Part model, mm, in its own coordinate system. A direction names the side the tool comes from. Give positions to 0.01 mm unless a question says otherwise; leave off trailing zeros. Write each loop counter-clockwise with the first axis right and the second up, starting at its lowest first coordinate (ties: lowest second). Pieces come first, ordered by that corner, then holes.
from build123d import *

# Parameters (mm, degrees)
BASE_EXTRUDE_THIN_DEPTH = 4.35
SKETCH2_W               = 1.8
SKETCH2_H               = 4.6
CUT_EXTRUDE1_DEPTH      = 36.373471698


with BuildPart() as part:
    # Sketch1 → Base-Extrude-Thin (new, symmetric)
    with BuildSketch(Plane(origin=(0, 0, 0), x_dir=(1, 0, 0), z_dir=(0, 1, 0))):
        with BuildLine():
            Line((-17.2, -7), (-17.2, -1.5))
            ThreePointArc((-17.2, -1.5), (-16.30105087, 0.420061486), (-14.250691112, 0.959292891))
            Line((-14.250691112, 0.959292891), (-9, 0))
            Line((-9, 0), (9, 0))
            Line((9, 0), (14.250691112, 0.959292891))
            ThreePointArc((14.250691112, 0.959292891), (16.30105087, 0.420061486), (17.2, -1.5))
            Line((17.2, -1.5), (17.2, -7))
            Line((17.2, -7), (16.7, -7))
            Line((16.7, -7), (16.7, -1.5))
            ThreePointArc((16.7, -1.5), (15.980840696, 0.036049189), (14.340552889, 0.467434313))
            Line((14.340552889, 0.467434313), (9.045299693, -0.5))
            Line((9.045299693, -0.5), (-9.045299693, -0.5))
            Line((-9.045299693, -0.5), (-14.340552889, 0.467434313))
            ThreePointArc((-14.340552889, 0.467434313), (-15.980840696, 0.036049189), (-16.7, -1.5))
            Line((-16.7, -1.5), (-16.7, -7))
            Line((-16.7, -7), (-17.2, -7))
        make_face()
    extrude(amount=BASE_EXTRUDE_THIN_DEPTH, both=True)

    # Sketch2 → Cut-Extrude1 (cut, through all)
    with BuildSketch(Plane(origin=(17.2, 0, 0), x_dir=(0, 0, -1), z_dir=(1, 0, 0))):
        with Locations((-4.5, 0)):
            Rectangle(SKETCH2_W, SKETCH2_H)
        with BuildLine():
            Line((-7, 2.35), (-7, -2.35))
            ThreePointArc((-7, -2.35), (-6.414213562, -3.764213562), (-5, -4.35))
            Line((-5, -4.35), (-5, -8))
            Line((-5, -8), (-10, -8))
            Line((-10, -8), (-10, 8))
            Line((-10, 8), (-5, 8))
            Line((-5, 8), (-5, 4.35))
            ThreePointArc((-5, 4.35), (-6.414213562, 3.764213562), (-7, 2.35))
        make_face()
    extrude(amount=-CUT_EXTRUDE1_DEPTH, mode=Mode.SUBTRACT)


solid = part.part
1) Mould opens along X. For faces 4 (the flat face through (-11.662, 0.061, -0.486)), 5 (the flat face through (-17.2, 0, 3)), 6 (the cylindrical face through (-15.962, 0.061, -0.052)), 7 (the flat face through (1.4, -4.35, 0.2)) say: +X half, -X half, draft (parallel to the pull), parting line (faces both ways), or undercut.
Check result:
face 4: undercut
face 5: -X half
face 6: undercut
face 7: draft
2) Saw through at A-A (z = 4). Write the cut outline in (x, y), and give its area (3 significant figures).
Check result:
outline: (-17.2, -4.35) - (-16.7, -4.35) - (-16.7, -2.3) - (-17.2, -2.3) - close; (-17.2, 2.3) - (-16.7, 2.3) - (-16.7, 4.35) - (-17.2, 4.35) - close; (16.7, -4.35) - (17.2, -4.35) - (17.2, -2.3) - (16.7, -2.3) - close; (16.7, 2.3) - (17.2, 2.3) - (17.2, 4.35) - (16.7, 4.35) - close
area: 4.10 mm2
3) Saw through at C-C (z = 2). Write the cut outline in (x, y), and give its area (3 significant figures).
Check result:
outline: (-17.2, -4.35) - (-16.7, -4.35) - (-16.7, 4.35) - (-17.2, 4.35) - close; (16.7, -4.35) - (17.2, -4.35) - (17.2, 4.35) - (16.7, 4.35) - close
area: 8.70 mm2
4) Flat gauge pins, fed straight in: P1, Ø4.5, axis at x = -2.5, y = 0, coming from the +Z side; P2, Ø2.5, axis at x = -2.5, y = 0, coming from the -Z side. Where does each tip first touch, or does it go through?
Check result:
P1: stops at z = 0.5
P2: stops at z = 0
5) Saw through at B-B (y = 0). Write the cut outline in (x, z).
Check result:
outline: (-17.2, 1.5) arc R2.5 ccw to (-14.25, -0.96) - (-9, 0) - (9, 0) - (14.25, -0.96) arc R2.5 ccw to (17.2, 1.5) - (17.2, 3.6) - (16.7, 3.6) - (16.7, 1.5) arc R2 cw to (14.34, -0.47) - (9.05, 0.5) - (-9.05, 0.5) - (-14.34, -0.47) arc R2 cw to (-16.7, 1.5) - (-16.7, 3.6) - (-17.2, 3.6) - close; (-17.2, 5.4) - (-16.7, 5.4) - (-16.7, 7) - (-17.2, 7) - close; (16.7, 5.4) - (17.2, 5.4) - (17.2, 7) - (16.7, 7) - close
6) 3-axis set-ups, long thin cutter, end or side, ignore diameter. For faces 1 (the flat face through (0, 0, 0)), 2 (the flat face through (16.7, 0, 3)), 3 (the flat face through (17.2, 0, 3)): which of +Z, -Z, +X, -X, +Y, -Y reach the whole face in a straight line?
Check result:
face 1: -Z, +Y, -Y
face 2: +Z, +Y, -Y
face 3: +Z, -Z, +X, +Y, -Y
7) Saw through at D-D (z = 6). Write the cut outline in (x, y), and give its area (3 significant figures).
Check result:
outline: (-17.2, -4.08) - (-16.7, -4.08) - (-16.7, 4.08) - (-17.2, 4.08) - close; (16.7, -4.08) - (17.2, -4.08) - (17.2, 4.08) - (16.7, 4.08) - close
area: 8.16 mm2
8) Drill centre lines: L1, parallel to X at y = -2.5, z = 4; L2, parallel to Z at x = -8, y = -3; L3, parallel to X at y = 2.5, z = 1. Where is each one in solid material? Low to high.
Check result:
L1: x = -17.2 to -16.7, 16.7 to 17.2
L2: z = 0 to 0.5
L3: x = -17.15 to -16.64, 16.64 to 17.15
